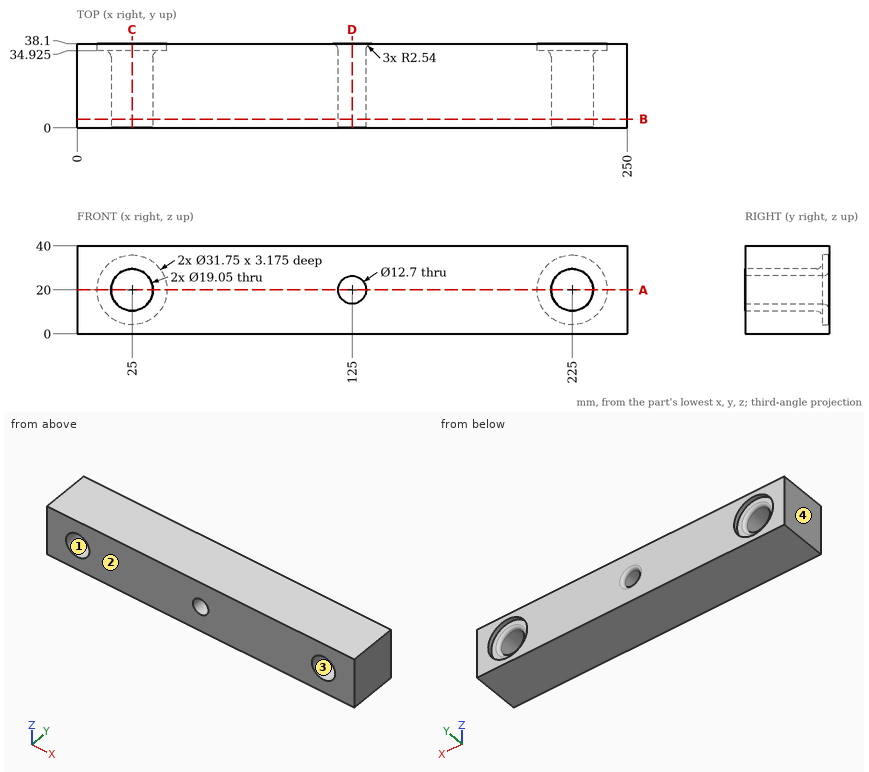
Verification items for this drawing (mm, ordinates from the low corner). Give positions to 0.01 mm unless a question says otherwise; leave off trailing zeros. Loops run counter-clockwise (first coordinate to the right, second up) from the corner with the lowest first, then second, coordinate; pieces in that order, holes last. Notation, with made-up numbers: M 50,11 L 57,11 A20 ccw 57,50 Z; hole C 17,34.25 d9. An arc over 180 degrees is marked long. Return JSON: item names as keys, results as strings. Group by question number.
1. Mould release check, pull along X, two halves, no side actions. Record for the marked faces 1, 2, 3 and 4: released by +X, released by -X, zero draft, split by the parting line, or undercut.
2. Cross-section at A-A on z = 20. State how many separate pieces and enclosed holes the cut face has, plus the area to 3 significant figures.
3. Cross-section at C-C on x = 25. Record the boundary of the cut face in (y, z) (3 decimals), plus the area to 3 significant figures.
4. Go/stop test with flat-tipped pins: pin 1 (12 mm diameter, centred on x = 130, z = 31.5, fed in from -Y); pin 2 (17 mm diameter, centred on x = 225, z = 20, fed in from +Y); pin 3 (16 mm diameter, centred on x = 27.5, z = 20.5, fed in from +Y). Record where each tip stops, or that it passes through.
5. Thickness scan on L1, parallel to X at y = 8, z = 20 (3 decimals); L2, parallel to X at y = 13, z = 24.5; L3, parallel to X at y = 4, z = 12.5. Record the ranges inside material, lowest first.
6. Cross-section at D-D on x = 125. Record the boundary of the cut face in (y, z), plus the area to 3 significant figures.
7. Cross-section at B-B on y = 4. Record the boundary of the cut face in (x, z) (3 decimals), plus the area to 3 significant figures.
Return value:
{
 "1": {"face 1": "undercut", "face 2": "zero draft", "face 3": "undercut", "face 4": "released by -X"},
 "2": {"separate pieces": "4", "enclosed holes": "0", "area": "7,500 mm^2"},
 "3": {"outline": "M 0,0 L 38.1,0 L 38.1,4.125 L 34.925,4.125 L 34.925,7.935 A2.54 ccw 32.385,10.475 L 0,10.475 Z; M 0,29.525 L 32.385,29.525 A2.54 ccw 34.925,32.065 L 34.925,35.875 L 38.1,35.875 L 38.1,40 L 0,40 Z", "area": "755 mm^2"},
 "4": {"pin 1": "y = 0", "pin 2": "through", "pin 3": "y = 34.42"},
 "5": {"L1": "0 to 15.475, 34.525 to 118.65, 131.35 to 215.475, 234.525 to 250", "L2": "0 to 16.61, 33.39 to 120.52, 129.48 to 216.61, 233.39 to 250", "L3": "0 to 19.13, 30.87 to 219.13, 230.87 to 250"},
 "6": {"outline": "M 0,0 L 38.1,0 L 38.1,11.11 A2.54 ccw 35.56,13.65 L 0,13.65 Z; M 0,26.35 L 35.56,26.35 A2.54 ccw 38.1,28.89 L 38.1,40 L 0,40 Z", "area": "1,040 mm^2"},
 "7": {"outline": "M 0,0 L 250,0 L 250,40 L 0,40 Z; hole C 25,20 d19.05; hole C 125,20 d12.7; hole C 225,20 d19.05", "area": "9,300 mm^2"}
}
